Geometry: final body of the model. Coordinates: model frame, mm. A direction names the side the tool comes from. Give positions to 0.01 mm unless a question says otherwise; leave off trailing zeros. Write each loop counter-clockwise with the first axis right and the second up, starting at its lowest first coordinate (ties: lowest second). Pieces come first, ordered by that corner, then holes. Notation, with made-up numbers: (37, -26) -> (90, -26) arc R16 ccw to (90, -5) -> close; hole circle Ø6 at (82.5, -36). An arc over 180 degrees is marked (long way). Answer in a Markdown table with one row per item. Add a question column.
Item 1: Section query D-D on x = -4. Output: boundary loops of the cut face in (y, z), plus the area to 3 significant figures.
Item 2: Material intervals for probe 1 along X at (y, z) = (2.5, -15.5); probe 2 along Y at (x, z) = (-5, -5); probe 3 along X at (y, z) = (2.5, -24), sorted ascending. Write a range as from..to.
Item 3: First-contact query: P1, Ø4, axis at y = -5, z = -5, coming from the -X side; P2, Ø5, axis at y = -6.5, z = 2.5, coming from the +X side; P3, Ø4, axis at x = 4, y = -3.5, coming from the +Z side; P4, Ø2, axis at y = -0.5, z = 14.5, coming from the +X side. Flat tips, straight axial feed; report the tip coordinate or a pass-through.
Item 4: Section query B-B on z = 5. State how many separate pieces and enclosed holes the cut face has, plus the area to 3 significant figures.
Item 5: Draft query along Y for faces 1 (the flat face through (-3, 2.8, -31)), 2 (the flat face through (-5, -10, 0)), 3 (the cylindrical face through (4.96, -6.22, -5.27)), 4 (the flat face through (7.5, -5, 0)). Return one class per face: +Y half, -Y half, draft (parallel to the pull), parting line (faces both ways), or undercut.
Item 6: Section query C-C on y = -5. Output: boundary loops of the cut face in (x, z).
Item 7: Section query A-A on y = -1.5. Output: boundary loops of the cut face in (x, z).
Item 8: Access query for faces 5 (the flat face through (-5, -5, 10)), 6 (the flat face through (-24.6, 1.676, 24.886)), 7 (the flat face through (-7.5, -5, 0)), 8 (the flat face through (-21.757, 2.496, -21.506)). Directions: +Z, -Z, +X, -X, +Y, -Y. A direction counts if a zero-diameter tool reaches every point of the face in a straight line with its end or side. Return the directions, or none.
Autodesk Inventor part; units mm, degrees
ref_plane "YZ Plane" through (0, 0, 0) normal (1, 0, 0) x (0, 1, 0)
ref_plane "XZ Plane" through (0, 0, 0) normal (0, 1, 0) x (-1, 0, 0)
ref_plane "XY Plane" through (0, 0, 0) normal (0, 0, 1) x (1, 0, 0)
sketch "스케치3" plane through (0, 0, 0) normal (0, 1, 0) x (-1, 0, 0)
  line L0 (34.9919, -14.4941) -> (14.4941, -34.9919)
  line L1 (14.4941, -34.9919) -> (-14.4941, -34.9919)
  line L2 (-14.4941, -34.9919) -> (-34.9919, -14.4941)
  line L3 (-34.9919, -14.4941) -> (-34.9919, 14.4941)
  line L4 (-34.9919, 14.4941) -> (-14.4941, 34.9919)
  line L5 (-14.4941, 34.9919) -> (14.4941, 34.9919)
  line L6 (14.4941, 34.9919) -> (34.9919, 14.4941)
  line L7 (34.9919, 14.4941) -> (34.9919, -14.4941)
  line L8 (13.5, -32.5919) -> (-13.5, -32.5919)
  line L9 (-13.5, -32.5919) -> (-32.5919, -13.5)
  line L10 (-32.5919, -13.5) -> (-32.5919, 13.5)
  line L11 (-32.5919, 13.5) -> (-13.5, 32.5919)
  line L12 (-13.5, 32.5919) -> (13.5, 32.5919)
  line L13 (13.5, 32.5919) -> (32.5919, 13.5)
  line L14 (32.5919, 13.5) -> (32.5919, -13.5)
  line L15 (32.5919, -13.5) -> (13.5, -32.5919)
  point P0 (0, 0)
  point P1 (0, 0)
  point P2 (0, 0)
  point P3 (0, 0)
  dimension "d66" = 27
  dimension "d67" = 2.4
extrude "돌출2" add sketch "스케치3" along normal blind 3.4 contours L0 L1 L2 L3 L4 L5 L6 L7 | L8 L9 L10 L11 L12 L13 L14 L15
sketch "스케치4" plane through (0, 3.4, 0) normal (0, 1, 0) x (1, 0, 0)
  line L0 (13.5, -32.5919) -> (-13.5, -32.5919)
  line L1 (-13.5, -32.5919) -> (-32.5919, -13.5)
  line L2 (-32.5919, -13.5) -> (-32.5919, 13.5)
  line L3 (-32.5919, 13.5) -> (-13.5, 32.5919)
  line L4 (-13.5, 32.5919) -> (13.5, 32.5919)
  line L5 (13.5, 32.5919) -> (32.5919, 13.5)
  line L6 (32.5919, 13.5) -> (32.5919, -13.5)
  line L7 (32.5919, -13.5) -> (13.5, -32.5919)
  line L8 (-13.9971, 33.7919) -> (13.9971, 33.7919)
  line L9 (13.9971, 33.7919) -> (33.7919, 13.9971)
  line L10 (33.7919, 13.9971) -> (33.7919, -13.9971)
  line L11 (33.7919, -13.9971) -> (13.9971, -33.7919)
  line L12 (13.9971, -33.7919) -> (-13.9971, -33.7919)
  line L13 (-13.9971, -33.7919) -> (-33.7919, -13.9971)
  line L14 (-33.7919, -13.9971) -> (-33.7919, 13.9971)
  line L15 (-33.7919, 13.9971) -> (-13.9971, 33.7919)
  line L16 (-13.1686, 31.7919) -> (13.1686, 31.7919)
  line L17 (13.1686, 31.7919) -> (31.7919, 13.1686)
  line L18 (31.7919, 13.1686) -> (31.7919, -13.1686)
  line L19 (31.7919, -13.1686) -> (13.1686, -31.7919)
  line L20 (13.1686, -31.7919) -> (-13.1686, -31.7919)
  line L21 (-13.1686, -31.7919) -> (-31.7919, -13.1686)
  line L22 (-31.7919, -13.1686) -> (-31.7919, 13.1686)
  line L23 (-31.7919, 13.1686) -> (-13.1686, 31.7919)
  point P0 (0, 0)
  point P1 (0, 0)
  point P2 (0, 0)
  point P3 (0, 0)
  dimension "d7" = 27
  dimension "d68" = 1.2
  dimension "d69" = 0.8
extrude "돌출3" cut sketch "스케치4" against normal blind 1.2 contours L0 L1 L2 L3 L4 L5 L6 L7 | L8 L9 L10 L11 L12 L13 L14 L15 | L16 L17 L18 L19 L20 L21 L22 L23
sketch "스케치9" plane through (0, 0, 0) normal (0, -1, 0) x (1, 0, 0)
  line L0 (7.5, 10) -> (2.5, 10)
  line L1 (2.5, 10) -> (2.5, -10)
  line L2 (2.5, -10) -> (7.5, -10)
  line L3 (7.5, -10) -> (7.5, 10)
  line L4 (7.5, 10) -> (2.5, -10) construction
  line L5 (2.5, 10) -> (7.5, -10) construction
  line L6 (-2.5, 10) -> (-7.5, 10)
  line L7 (-7.5, 10) -> (-7.5, -10)
  line L8 (-7.5, -10) -> (-2.5, -10)
  line L9 (-2.5, 10) -> (-7.5, -10) construction
  line L10 (-7.5, 10) -> (-2.5, -10) construction
  line L11 (-2.5, -10) -> (-2.5, 10)
  point P0 (0, 0)
  point P1 (5, 0)
  point P2 (-5, 0)
  dimension "d42" = 20
  dimension "d43" = 5
  dimension "d44" = 2.5
  dimension "d47" = 10
extrude "돌출8" add sketch "스케치9" along normal blind 10
sketch "스케치10" plane through (-7.5, 0, -10) normal (-1, 0, 0) x (0, 0, 1)
  circle A0 centre (15, -5) radius 1.25
  line L0 (19.9591, 0) -> (0.0886, 0)
  line L1 (24.4941, 0) -> (-4.4941, 0)
  circle A1 centre (5, -5) radius 1.25
  line L2 (20, 0) -> (20, -10)
  point P0 (10, 0)
  dimension "d54" = 2.5
  dimension "d57" = 10
  dimension "d62" = 5
  dimension "d63" = 5
extrude "돌출9" cut sketch "스케치10" against normal blind 20
sketch "스케치11" plane through (0, 2.2, 0) normal (0, 1, 0) x (1, 0, 0)
  line L0 (-13.1686, 31.7919) -> (13.1686, 31.7919)
  line L1 (13.1686, 31.7919) -> (31.7919, 13.1686)
  line L2 (31.7919, 13.1686) -> (31.7919, -13.1686)
  line L3 (31.7919, -13.1686) -> (13.1686, -31.7919)
  line L4 (13.1686, -31.7919) -> (-13.1686, -31.7919)
  line L5 (-13.1686, -31.7919) -> (-31.7919, -13.1686)
  line L6 (-31.7919, -13.1686) -> (-31.7919, 13.1686)
  line L7 (-31.7919, 13.1686) -> (-13.1686, 31.7919)
  line L8 (-13.9971, 33.7919) -> (13.9971, 33.7919)
  line L9 (-12.6716, 30.5919) -> (12.6716, 30.5919)
  line L10 (12.6716, 30.5919) -> (30.5919, 12.6716)
  line L11 (30.5919, 12.6716) -> (30.5919, -12.6716)
  line L12 (30.5919, -12.6716) -> (12.6716, -30.5919)
  line L13 (12.6716, -30.5919) -> (-12.6716, -30.5919)
  line L14 (-12.6716, -30.5919) -> (-30.5919, -12.6716)
  line L15 (-30.5919, -12.6716) -> (-30.5919, 12.6716)
  line L16 (-30.5919, 12.6716) -> (-12.6716, 30.5919)
  point P0 (0, 0)
  point P1 (0, 0)
  point P2 (0, 0)
  dimension "d70" = 2
  dimension "d71" = 1.2
extrude "돌출10" add sketch "스케치11" along normal blind 0.6
properties part number "팔각형 OV-PAM 5패턴 하단 - 틈 너비 수정"
Findings below:
| question | item | result |
|---|---|---|
| 1 | outline | (-10, -10) -> (0, -10) -> (0, -34.99) -> (3.4, -34.99) -> (3.4, -33.79) -> (2.2, -33.79) -> (2.2, -31.79) -> (2.8, -31.79) -> (2.8, -30.59) -> (2.2, -30.59) -> (2.2, 30.59) -> (2.8, 30.59) -> (2.8, 31.79) -> (2.2, 31.79) -> (2.2, 33.79) -> (3.4, 33.79) -> (3.4, 34.99) -> (0, 34.99) -> (0, 10) -> (-10, 10) -> close; hole circle Ø2.5 at (-5, -5); hole circle Ø2.5 at (-5, 5) |
| 1 | area | 348 mm^2 |
| 2 | probe 1 | x = -33.99..-32.29, -29.46..-27.76, 27.76..29.46, 32.29..33.99 |
| 2 | probe 2 | y = -10..-6.25, -3.75..2.2 |
| 2 | probe 3 | x = -25.49..-23.79, -20.96..-19.26, 19.26..20.96, 23.79..25.49 |
| 3 | P1 | stops at x = -7.5 |
| 3 | P2 | stops at x = 7.5 |
| 3 | P3 | stops at z = 10 |
| 3 | P4 | stops at x = 34.99 |
| 4 | separate pieces | 3 |
| 4 | enclosed holes | 0 |
| 4 | area | 233 mm^2 |
| 5 | face 1 | +Y half |
| 5 | face 2 | -Y half |
| 5 | face 3 | undercut |
| 5 | face 4 | draft |
| 6 | outline | (-7.5, -10) -> (-2.5, -10) -> (-2.5, -6.25) -> (-7.5, -6.25) -> close; (-7.5, -3.75) -> (-2.5, -3.75) -> (-2.5, 3.75) -> (-7.5, 3.75) -> close; (-7.5, 6.25) -> (-2.5, 6.25) -> (-2.5, 10) -> (-7.5, 10) -> close; (2.5, -10) -> (7.5, -10) -> (7.5, -6.25) -> (2.5, -6.25) -> close; (2.5, -3.75) -> (7.5, -3.75) -> (7.5, 3.75) -> (2.5, 3.75) -> close; (2.5, 6.25) -> (7.5, 6.25) -> (7.5, 10) -> (2.5, 10) -> close |
| 7 | outline | (-7.5, -10) -> (-2.5, -10) -> (-2.5, 10) -> (-7.5, 10) -> close; (2.5, -10) -> (7.5, -10) -> (7.5, 10) -> (2.5, 10) -> close |
| 8 | face 5 | +Z, +X, -X, -Y |
| 8 | face 6 | +Z, -X, +Y, -Y |
| 8 | face 7 | +Z, -Z, -X, -Y |
| 8 | face 8 | +Y |
